```python
from build123d import *

# Parameters (mm, degrees)
SKETCH1_W           = 450
SKETCH1_H           = 20
BOSS_EXTRUDE1_DEPTH = 800
CUT_EXTRUDE1_DEPTH  = 919.095855562


with BuildPart() as part:
    # Sketch1 → Boss-Extrude1 (new body)
    with BuildSketch(Plane.XY):
        with Locations((-225, 10)):
            Rectangle(SKETCH1_W, SKETCH1_H)
    extrude(amount=BOSS_EXTRUDE1_DEPTH)

    # Sketch2 → Cut-Extrude1 (cut, through all)
    with BuildSketch(Plane.XY.offset(800)):
        Polygon((-430, 20), (-430, 13.5), (-433, 13.5), (-433, 5.5), (-417, 5.5), (-417, 13.5), (-420, 13.5), (-420, 20), align=None)
        Polygon((-380, 20), (-380, 13.5), (-383, 13.5), (-383, 5.5), (-367, 5.5), (-367, 13.5), (-370, 13.5), (-370, 20), align=None)
        Polygon((-330, 20), (-330, 13.5), (-333, 13.5), (-333, 5.5), (-317, 5.5), (-317, 13.5), (-320, 13.5), (-320, 20), align=None)
        Polygon((-280, 20), (-280, 13.5), (-283, 13.5), (-283, 5.5), (-267, 5.5), (-267, 13.5), (-270, 13.5), (-270, 20), align=None)
        Polygon((-230, 20), (-230, 13.5), (-233, 13.5), (-233, 5.5), (-217, 5.5), (-217, 13.5), (-220, 13.5), (-220, 20), align=None)
        Polygon((-180, 20), (-180, 13.5), (-183, 13.5), (-183, 5.5), (-167, 5.5), (-167, 13.5), (-170, 13.5), (-170, 20), align=None)
        Polygon((-130, 20), (-130, 13.5), (-133, 13.5), (-133, 5.5), (-117, 5.5), (-117, 13.5), (-120, 13.5), (-120, 20), align=None)
        Polygon((-80, 20), (-80, 13.5), (-83, 13.5), (-83, 5.5), (-67, 5.5), (-67, 13.5), (-70, 13.5), (-70, 20), align=None)
        Polygon((-30, 20), (-30, 13.5), (-33, 13.5), (-33, 5.5), (-17, 5.5), (-17, 13.5), (-20, 13.5), (-20, 20), align=None)
        Polygon((20, 20), (20, 13.5), (17, 13.5), (17, 5.5), (33, 5.5), (33, 13.5), (30, 13.5), (30, 20), align=None)
    extrude(amount=-CUT_EXTRUDE1_DEPTH, mode=Mode.SUBTRACT)


solid = part.part
```
The listing builds one solid part. Answer for the finished solid, in the listing's coordinates (mm). A direction names the side the tool comes from. Coordinates: 2 decimals unless noted, no trailing zeros. Return JSON: item names as keys, results as strings. Group by question number.
1. Which of the six approach directions +Z, -Z, +X, -X, +Y, -Y give full straight-line access (tool end or side, diameter ignored) to faces 3 (the flat face through (-200, 20, 394)), 4 (the flat face through (-175, 5.5, 406))?
2. Straight lines are drawn through the part: L1, parallel to Y at x = -232, z = 612.5; L2, parallel to Y at x = -179.5, z = 34. For each, find the intervals that lie inside material, in ascending order.
3. Determine the mould class of faces 1 (the flat face through (-226, 5, 800)), 2 (the flat face through (-275, 5.5, 406)) for opening direction X: released by +X, released by -X, zero draft, split by the parting line, or undercut.
4. A cutting plane is placed at A-A, the plane y = 9. Give the number of separate pieces and of enclosed holes in the cut face, plus the area to 3 significant figures.
Ans:
{
 "1": {"face 3": "+Z, -Z, +X, -X, +Y", "face 4": "+Z, -Z"},
 "2": {"L1": "0 to 5.5, 13.5 to 20", "L2": "0 to 5.5"},
 "3": {"face 1": "zero draft", "face 2": "undercut"},
 "4": {"separate pieces": "10", "enclosed holes": "0", "area": "245,000 mm²"}
}
